Part model, mm, in its own coordinate system. Face numbers are marked on the shaded views. Coordinates: 2 decimals unless noted, no trailing zeros. Write each loop counter-clockwise with the first axis right and the second up, starting at its lowest first coordinate (ties: lowest second). Pieces come first, ordered by that corner, then holes. Notation, with made-up numbers: (1, 14.25) -> (26, 14.25) arc R24 ccw to (26, 52.25) -> close; hole circle Ø11 at (59.25, -13). An arc over 180 degrees is marked (long way). Write item = value, one per line. Start each with the question number.
Q1. Band-saw the part on D-D, the plane y = 5. List the corners of the cut face in (x, z), plus the area to 3 significant figures.
Q2. Band-saw the part on A-A, the plane z = 0. List the corners of the cut face in (x, y).
Q3. Probe line 1 (X direction, y = 7, z = 0); line 2 (X direction, y = 14, z = 0); line 3 (X direction, y = 3, z = -0.5). List the from-to ranges inside material, lowest first.
Q4. Band-saw the part on C-C, the plane x = -2.25. List the corners of the cut face in (y, z), plus the area to 3 significant figures.
Q5. Band-saw the part on B-B, the plane y = 20. List the corners of the cut face in (x, z), plus the area to 3 significant figures.
Q6. Pin check, flat tips, straight feed: P1, Ø3, axis at y = 27, z = 2.5, coming from the -X side; P2, Ø1.5, axis at x = 0.5, z = -0.5, coming from the -Y side. Stop position of each tip, or through.
Q7. Pull direction Z, two halves, no side cores. Call the marked faces 1, 2 and 3: released by +Z, released by -Z, zero draft, split by the parting line, or undercut.
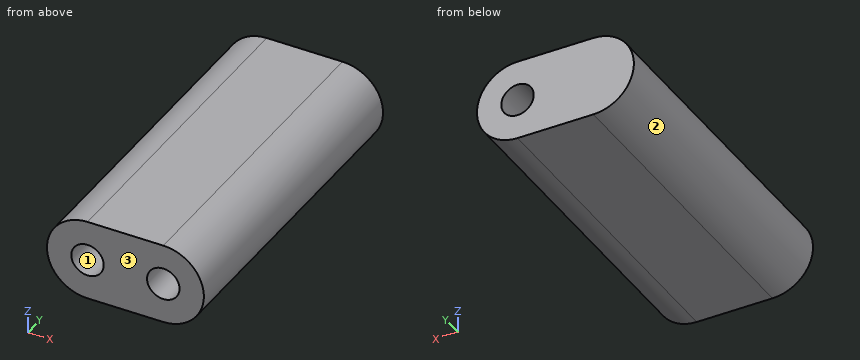
from build123d import *

# Parameters (mm, degrees)
BOSS_EXTRUDE2_DEPTH = 30
SKETCH2_R           = 1.5
CUT_EXTRUDE1_DEPTH  = 30
SKETCH3_R           = 1.5
CUT_EXTRUDE2_DEPTH  = 10


with BuildPart() as part:
    # Sketch1 → Boss-Extrude2 (new body)
    with BuildSketch(Plane(origin=(0, 0, 0), x_dir=(1, 0, 0), z_dir=(0, 1, 0))):
        with BuildLine():
            ThreePointArc((0, 3.75), (-3.75, 0), (0, -3.75))
            Line((0, -3.75), (7, -3.75))
            ThreePointArc((7, -3.75), (10.75, 0), (7, 3.75))
            Line((7, 3.75), (0, 3.75))
        make_face()
    extrude(amount=BOSS_EXTRUDE2_DEPTH)

    # Sketch2 → Cut-Extrude1 (cut)
    with BuildSketch(Plane(origin=(0, 30, 0), x_dir=(1, 0, 0), z_dir=(0, 1, 0))):
        with Locations(Location((7, 0, 0), (0, 0, 270))):
            Circle(SKETCH2_R)
    extrude(amount=-CUT_EXTRUDE1_DEPTH, mode=Mode.SUBTRACT)

    # Sketch3 → Cut-Extrude2 (cut)
    with BuildSketch(Plane.XZ):
        with Locations(Location((0, 0, 0), (0, 0, 270))):
            Circle(SKETCH3_R)
    extrude(amount=-CUT_EXTRUDE2_DEPTH, mode=Mode.SUBTRACT)


solid = part.part
Ans:
q1.outline = (0, -3.75) -> (7, -3.75) arc R3.75 ccw to (7, 3.75) -> (0, 3.75) arc R3.75 ccw to start; hole circle Ø3 at (0, 0); hole circle Ø3 at (7, 0)
q1.area = 82.5 mm2
q2.outline = (-3.75, 0) -> (-1.5, 0) -> (-1.5, 10) -> (1.5, 10) -> (1.5, 0) -> (5.5, 0) -> (5.5, 30) -> (-3.75, 30) -> close; (8.5, 0) -> (10.75, 0) -> (10.75, 30) -> (8.5, 30) -> close
q3.line_1 = -3.75 to -1.5, 1.5 to 5.5, 8.5 to 10.75
q3.line_2 = -3.75 to 5.5, 8.5 to 10.75
q3.line_3 = -3.72 to -1.41, 1.41 to 5.59, 8.41 to 10.72
q4.outline = (0, -3) -> (30, -3) -> (30, 3) -> (0, 3) -> close
q4.area = 180 mm2
q5.outline = (0, -3.75) -> (7, -3.75) arc R3.75 ccw to (7, 3.75) -> (0, 3.75) arc R3.75 ccw to start; hole circle Ø3 at (7, 0)
q5.area = 89.6 mm2
q6.P1 = -3.61
q6.P2 = 10
q7.face_1 = undercut
q7.face_2 = split by the parting line
q7.face_3 = zero draft
